The model under review builds one solid part; all positions refer to its coordinate system, in mm. A direction names the side the tool comes from. Round coordinates to 2 decimals unless told otherwise and drop trailing zeros. Write each loop counter-clockwise with the first axis right and the second up, starting at its lowest first coordinate (ties: lowest second). Pieces come first, ordered by that corner, then holes. Notation, with made-up numbers: (42, 79.25) -> (51, 79.25) arc R20 cw to (51, 115.25) -> close; hole circle Ø11 at (23, -21.5). An arc over 180 degrees is marked (long way). Return JSON: item names as keys, results as strings. Group by question number.
1. Clearance check with flat-ended pins moving along their axes: P1, Ø4, axis at x = 23.5, y = 4.5, coming from the -Z side; P2, Ø6, axis at x = 27.5, y = 2, coming from the +Z side; P3, Ø4, axis at x = 2.5, z = 3, coming from the -Y side. State where each tip first meets the part, or that it passes through.
2. Take a section at A-A, the plane x = -17.5. Write out the cut boundary in (y, z).
3. Tool access review of faces 1 (the flat face through (45, 9, 0)), 2 (the cylindrical face through (3.31, -1.08, -4.88)): name each direction out of +Z, -Z, +X, -X, +Y, -Y from which nothing blocks a thin tool from reaching the whole face with its end or side.
4. For line 1 along X through (y, z) = (-2.75, -6.5); line 2 along Z through (x, y) = (-18.5, -2.25); line 3 along X through (y, z) = (7.5, 5.5), list the stretches that pass through material, from the lowest coordinate up. Write a range as from..to.
from build123d import *

# Parameters (mm, degrees)
SKETCH4_W           = 18
SKETCH4_H           = 18
BOSS_EXTRUDE1_DEPTH = 8
SKETCH5_OUTSIDE_W   = 72.14
SKETCH5_OUTSIDE_H   = 72.14
SKETCH5_OUTSIDE_R   = 9
CUT_EXTRUDE3_DEPTH  = 10
CUT_EXTRUDE3_TAPER  = 60


with BuildPart() as part:
    # Sketch1 → Revolve1 (revolve)
    with BuildSketch(Plane.XY):
        Polygon((-33.667489974, 5), (-34.374596755, 4.292893219), (-34.374596755, 0), (41.332510026, 0), (41.332510026, 5), align=None)
    revolve(axis=Axis((-59.973351377, 0, 0), (1, 0, 0)))

    # Sketch4 → Boss-Extrude1 (add)
    with BuildSketch(Plane(origin=(41.332510026, 0, 0), x_dir=(0, 0, -1), z_dir=(1, 0, 0))):
        Rectangle(SKETCH4_W, SKETCH4_H)
    extrude(amount=BOSS_EXTRUDE1_DEPTH)

    # Sketch5 outside → Cut-Extrude3 (cut)
    with BuildSketch(Plane(origin=(49.332510026, 0, 0), x_dir=(0, 0, -1), z_dir=(1, 0, 0))):
        Rectangle(SKETCH5_OUTSIDE_W, SKETCH5_OUTSIDE_H)
        Circle(SKETCH5_OUTSIDE_R, mode=Mode.SUBTRACT)
    extrude(amount=-CUT_EXTRUDE3_DEPTH, taper=CUT_EXTRUDE3_TAPER, mode=Mode.SUBTRACT)


solid = part.part
Output:
{
 "1": {"P1": "stops at z = -4.33", "P2": "stops at z = 5", "P3": "stops at y = -4.9"},
 "2": {"outline": "circle Ø10 at (0, 0)"},
 "3": {"face 1": "+Z, -Z, +X, -X, +Y", "face 2": "-X"},
 "4": {"line 1": "x = 41.33..49.33", "line 2": "z = -4.47..4.47", "line 3": "x = 41.33..49.16"}
}
